Verification items for the finished model (mm, model axes). Coordinates: 2 decimals unless noted, no trailing zeros. Order: outer loops, then holes, each group sorted by start corner. A loop starts at its lowest first (then second) coordinate and runs counter-clockwise, first axis right, second up. Notation, with made-up numbers: (10, -38.5) - (22, -38.5) arc R15 ccw to (22, -14.5) - close; hole circle Ø6 at (-11, 80.5). An arc over 180 degrees is marked (long way). Answer as CSV lines item,"result". Start each with the question number.
1. Section check A-A (x = 75). Record the cut outline in (y, z), and give its area (3 significant figures).
2. Material ranges on L1, parallel to X at y = -269.5, z = 5.7; L2, parallel to Y at x = 265, z = 2; L3, parallel to Y at x = 2, z = 4.4, recorded low to high. Write a range as [from, to].
3. Section check B-B (y = -178.5). Record the cut outline in (x, z), and give its area (3 significant figures).
4. Section check D-D (z = 4.3). Count the separate pieces of the cut face and the enclosed holes in it, and give its area (3 significant figures).
5. Section check C-C (x = 144). Record the cut outline in (y, z).
6. Go/stop test with flat-tipped pins: pin 1 (1.8 mm diameter, centred on x = 146, z = 3, fed in from +Y); pin 2 (3 mm diameter, centred on x = 146.5, z = 3.5, fed in from -Y); pin 3 (1 mm diameter, centred on y = -271, z = 1, fed in from +X). Record where each tip stops, or that it passes through.
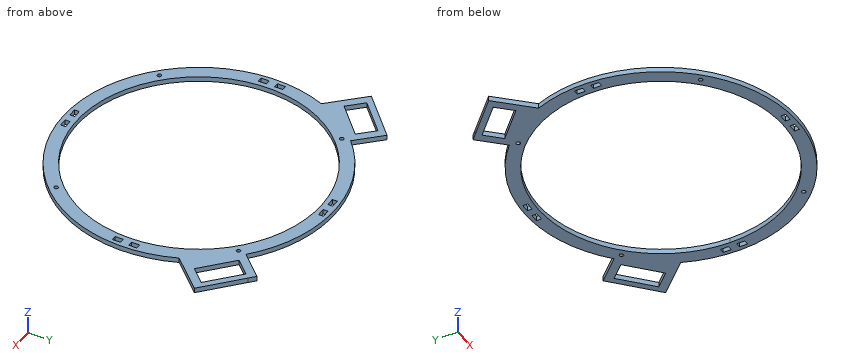
from build123d import *

# Parameters (mm, degrees)
SALIENTE_EXTRUIR1_DEPTH = 6
CROQUIS2_W              = 10
CROQUIS2_H              = 6
CROQUIS2_W_2            = 6
CROQUIS2_H_2            = 10
CORTAR_EXTRUIR1_DEPTH   = 10


with BuildPart() as part:
    # Croquis1 → Saliente-Extruir1 (new body)
    with BuildSketch(Plane.XY):
        with BuildLine():
            ThreePointArc((267.780622857, -36.999917491), (154.190797134, 7.728122029), (40.600971411, -36.999917491))
            Line((40.600971411, -36.999917491), (13.169180469, -7.88811841))
            Line((13.169180469, -7.88811841), (5.891230699, -14.746066146))
            Line((5.891230699, -14.746066146), (-37.776467922, -55.893752559))
            Line((-37.776467922, -55.893752559), (-0.057755376, -95.922476295))
            ThreePointArc((-0.057755376, -95.922476295), (154.190797134, -325.468820804), (308.439349644, -95.922476295))
            Line((308.439349644, -95.922476295), (346.15806219, -55.893752559))
            Line((346.15806219, -55.893752559), (302.490363569, -14.746066146))
            Line((302.490363569, -14.746066146), (295.212413799, -7.88811841))
            Line((295.212413799, -7.88811841), (267.780622857, -36.999917491))
        make_face()
        with BuildLine():
            ThreePointArc((50.939396199, -50.062499464), (51.321581101, -49.701102835), (51.705030941, -49.341048614))
            ThreePointArc((51.705030941, -49.341048614), (213.886421224, -21.26063874), (304.190797134, -158.870349387))
            ThreePointArc((304.190797134, -158.870349387), (94.978087942, -296.688545102), (50.939396199, -50.062499464))
        make_face(mode=Mode.SUBTRACT)
        Polygon((-25.35505735, -54.494267151), (11.034691501, -20.204528474), (28.17956084, -38.399402899), (-8.210188011, -72.689141577), align=None, mode=Mode.SUBTRACT)
        Polygon((316.591782279, -72.689141577), (280.202033428, -38.399402899), (297.346902767, -20.204528474), (333.736651618, -54.494267151), align=None, mode=Mode.SUBTRACT)
    extrude(amount=SALIENTE_EXTRUIR1_DEPTH)

    # Croquis2 → Cortar-Extruir1 (cut)
    with BuildSketch(Plane.XY.offset(6)):
        Polygon((139.190797134, -3.571113679), (149.190797134, -3.571113679), (149.190797134, -0.571113679), (149.190797134, 2.428886321), (139.190797134, 2.428886321), align=None)
        with Locations((164.190797134, -0.571113679)):
            Rectangle(CROQUIS2_W, CROQUIS2_H)
        with Locations((312.490032842, -148.870349387)):
            Rectangle(CROQUIS2_W_2, CROQUIS2_H_2)
        Polygon((312.490032842, -163.870349387), (315.490032842, -163.870349387), (315.490032842, -173.870349387), (309.490032842, -173.870349387), (309.490032842, -163.870349387), align=None)
        with Locations((164.190797134, -317.169585095)):
            Rectangle(CROQUIS2_W, CROQUIS2_H)
        Polygon((149.190797134, -317.169585095), (149.190797134, -314.169585095), (139.190797134, -314.169585095), (139.190797134, -320.169585095), (149.190797134, -320.169585095), align=None)
        with Locations((-4.108438574, -148.870349387)):
            Rectangle(CROQUIS2_W_2, CROQUIS2_H_2)
        Polygon((-7.108438574, -173.870349387), (-7.108438574, -163.870349387), (-4.108438574, -163.870349387), (-1.108438574, -163.870349387), (-1.108438574, -173.870349387), align=None)
        with BuildLine():
            ThreePointArc((40.506244825, -45.185797078), (40.506244825, -48.685975645), (44.006423391, -48.685975645))
            Line((44.006423391, -48.685975645), (40.506244825, -45.185797078))
        make_face()
        with BuildLine():
            Line((40.506244825, -45.185797078), (44.006423391, -48.685975645))
            ThreePointArc((44.006423391, -48.685975645), (44.542935951, -47.883027856), (44.731334108, -46.935886361))
            ThreePointArc((44.731334108, -46.935886361), (43.203475603, -44.649284518), (40.506244825, -45.185797078))
        make_face()
        with BuildLine():
            ThreePointArc((267.875349443, -45.185797078), (264.375170876, -45.185797078), (264.375170876, -48.685975645))
            Line((264.375170876, -48.685975645), (267.875349443, -45.185797078))
        make_face()
        with BuildLine():
            Line((267.875349443, -45.185797078), (264.375170876, -48.685975645))
            ThreePointArc((264.375170876, -48.685975645), (267.072401655, -49.222488204), (268.60026016, -46.935886361))
            ThreePointArc((268.60026016, -46.935886361), (268.411862003, -45.988744866), (267.875349443, -45.185797078))
        make_face()
        with BuildLine():
            ThreePointArc((268.60026016, -270.804812413), (267.072401655, -268.51821057), (264.375170876, -269.05472313))
            Line((264.375170876, -269.05472313), (267.875349443, -272.554901696))
            ThreePointArc((267.875349443, -272.554901696), (268.411862003, -271.751953908), (268.60026016, -270.804812413))
        make_face()
        with BuildLine():
            Line((267.875349443, -272.554901696), (264.375170876, -269.05472313))
            ThreePointArc((264.375170876, -269.05472313), (264.375170876, -272.554901696), (267.875349443, -272.554901696))
        make_face()
        with BuildLine():
            ThreePointArc((44.731334108, -270.804812413), (44.542935951, -269.857670918), (44.006423391, -269.05472313))
            Line((44.006423391, -269.05472313), (40.506244825, -272.554901696))
            ThreePointArc((40.506244825, -272.554901696), (43.203475603, -273.091414256), (44.731334108, -270.804812413))
        make_face()
        with BuildLine():
            Line((40.506244825, -272.554901696), (44.006423391, -269.05472313))
            ThreePointArc((44.006423391, -269.05472313), (40.506244825, -269.05472313), (40.506244825, -272.554901696))
        make_face()
    extrude(amount=-CORTAR_EXTRUIR1_DEPTH, mode=Mode.SUBTRACT)


solid = part.part
Evaluation:
1,outline,"(-305.44, 0) - (-286.26, 0) - (-286.26, 6) - (-305.44, 6) - close; (-31.48, 0) - (-12.3, 0) - (-12.3, 6) - (-31.48, 6) - close"
1,area,"230 mm²"
2,L1,"x = [29.63, 40.15], [44.36, 52.89], [255.49, 264.02], [268.23, 278.75]"
2,L2,"y = [-283.27, -273.01], [-268.6, -259.97], [-57.77, -49.14], [-44.73, -34.47]"
2,L3,"y = [-226.64, -63.07], [-28.72, -18.41]"
3,outline,"(-11.25, 0) - (5.48, 0) - (5.48, 6) - (-11.25, 6) - close; (302.9, 0) - (319.63, 0) - (319.63, 6) - (302.9, 6) - close"
3,area,"201 mm²"
4,separate pieces,"1"
4,enclosed holes,"15"
4,area,"19,700 mm²"
5,outline,"(-325.16, 0) - (-320.17, 0) - (-320.17, 6) - (-325.16, 6) - close; (-314.17, 0) - (-308.52, 0) - (-308.52, 6) - (-314.17, 6) - close; (-9.22, 0) - (-3.57, 0) - (-3.57, 6) - (-9.22, 6) - close; (2.43, 0) - (7.42, 0) - (7.42, 6) - (2.43, 6) - close"
6,pin 1,"stops at y = 7.57"
6,pin 2,"stops at y = -325.35"
6,pin 3,"stops at x = 277.86"
